from build123d import *

# Parameters (mm, degrees)
F1_DEPTH = 63.5
F0_W     = 25.4
F0_H     = 19.05
F2_DEPTH = 25.4
F3_DEPTH = 7.9375


with BuildPart() as f1:
    # F0 (on Front) → F1 (new body, symmetric)
    with BuildSketch(Plane.XZ):
        Polygon((22.225, 9.525), (-41.275, 9.525), (-41.275, -9.525), (41.275, -9.525), (41.275, 9.525), align=None)
    extrude(amount=F1_DEPTH, both=True)

    # F0 (on Front) → F2 (join, symmetric)
    with BuildSketch(Plane.XZ):
        with BuildLine():
            Line((22.225, 25.4), (22.225, 9.525))
            Line((22.225, 9.525), (41.275, 9.525))
            Line((41.275, 9.525), (41.275, 25.4))
            ThreePointArc((41.275, 25.4), (45.9246798487, 36.6253201513), (57.15, 41.275))
            Line((57.15, 41.275), (60.325, 41.275))
            Line((60.325, 41.275), (60.325, 60.325))
            Line((60.325, 60.325), (57.15, 60.325))
            add(Edge.make_bspline(
                [(54.4736162544, 60.222300255), (55.3644540215, 60.2602361648), (56.2566409869, 60.2943854647), (57.15, 60.325)],
                knots=[108.3462442053, 108.3462442053, 108.3462442053, 108.3462442053, 110.761548495, 110.761548495, 110.761548495, 110.761548495], degree=3))
            ThreePointArc((54.4736162544, 60.222300255), (31.5255163241, 49.1306017906), (22.225, 25.4))
        make_face()
        with Locations((73.025, 50.8)):
            Rectangle(F0_W, F0_H)
    extrude(amount=F2_DEPTH, both=True)

    # F0 (on Front) → F3 (join, symmetric)
    with BuildSketch(Plane.XZ):
        with BuildLine():
            add(Edge.make_bspline(
                [(-41.275, 9.525), (-22.7342342872, 49.1991834723), (14.5122222919, 58.5205629773), (54.4736162544, 60.222300255)],
                knots=[0, 0, 0, 0, 108.3462442053, 108.3462442053, 108.3462442053, 108.3462442053], degree=3))
            Line((-41.275, 9.525), (22.225, 9.525))
            Line((22.225, 9.525), (22.225, 25.4))
            ThreePointArc((22.225, 25.4), (31.5255163241, 49.1306017906), (54.4736162544, 60.222300255))
        make_face()
    extrude(amount=F3_DEPTH, both=True)

    # F0 (on Front) → F4 (revolve)
    with BuildSketch(Plane.XZ):
        Polygon((85.725, 66.675), (85.725, 60.325), (85.725, 41.275), (85.725, 38.1), (111.125, 38.1), (111.125, 66.675), align=None)
    revolve(axis=Axis((85.725, 0, 53.975), (0, 0, -1)))


solid = f1.part
Work out the finished part from the listing and answer in its coordinate system (mm). A direction names the side the tool comes from. Coordinates: 2 decimals unless noted, no trailing zeros. Write each loop counter-clockwise with the first axis right and the second up, starting at its lowest first coordinate (ties: lowest second). Pieces come first, ordered by that corner, then holes. Notation, with made-up numbers: (43, -20.75) - (87, -20.75) arc R19 cw to (87, -3.75) - close; hole circle Ø6 at (-30, -1). An arc over 180 degrees is marked (long way). One line per question, with ' | ' between items.
1) Find section B-B, the plane y = -55. Determine the outline of the cut face in (x, z) (3 decimals), and give its area (3 significant figures).
Checks:
outline: (-41.275, -9.525) - (41.275, -9.525) - (41.275, 9.525) - (-41.275, 9.525) - close | area: 1,570 mm2
2) For faces 5 (the face through (46, 25.4, 41)), 6 (the face through (60, -2, 60.325)), 7 (the face through (46, -25.4, 41)), 8 (the face through (22.225, -17, 18)), 9 (the face through (1, 35, 9.525)), determine the directions among +Z, -Z, +X, -X, +Y, -Y from which every point of the face is accessible in a straight line to the end or side of a thin tool.
Checks:
face 5: +Z, +X, -X, +Y | face 6: +Z, -X | face 7: +Z, +X, -X, -Y | face 8: +Z, -X, -Y | face 9: +Z, -X, +Y
3) Flat-ended cylindrical pins translate along their axes: P1, Ø3, axis at x = -11, z = 14.5, coming from the -Y side; P2, Ø3, axis at y = 12, z = 57, coming from the +X side; P3, Ø17.5, axis at y = 17.5, z = 20, coming from the -X side (3 decimals); P4, Ø17.5, axis at y = -19.5, z = 16, coming from the -X side (3 decimals). Find the tip coordinate at first contact, or state that the pin passes through.
Checks:
P1: y = -7.94 | P2: x = 108.85 | P3: x = 22.225 | P4: x = -41.275
4) Find section A-A, the plane z = -3. Determine the outline of the cut face in (x, y) (3 decimals).
Checks:
outline: (-41.275, -63.5) - (41.275, -63.5) - (41.275, 63.5) - (-41.275, 63.5) - close
5) Consider probe 1 along X at (y, z) = (37.5, 2.5) (3 decimals); probe 2 along Z at (x, y) = (-25, -54) (3 decimals); probe 3 along Y at (x, z) = (14.5, 13.5). Determine where each line is inside the solid, lowest interval first. Write a range as [from, to].
Checks:
probe 1: [-41.275, 41.275] | probe 2: [-9.525, 9.525] | probe 3: [-7.94, 7.94]
6) The mould has two halves that part along X. Classify faces 1 (the face through (45.8, -0.4, 36.5)), 2 (the face through (-41.275, -1, 0)), 3 (the face through (-1, 63.5, 0)), 4 (the face through (60, 2, 41.275)): +X half, -X half, draft (parallel to the pull), parting line (faces both ways), or undercut.
Checks:
face 1: undercut | face 2: -X half | face 3: draft | face 4: undercut
